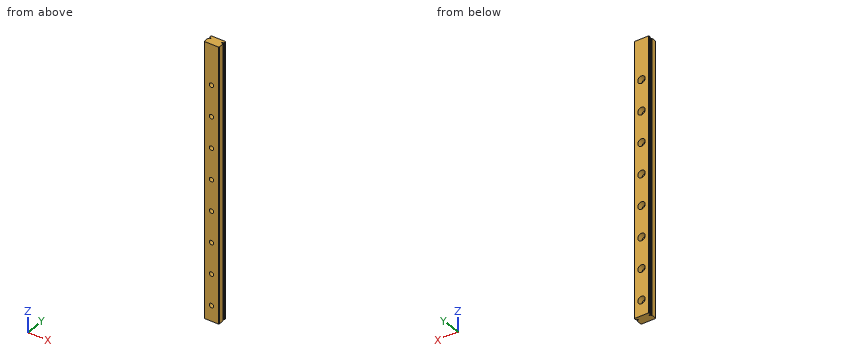
from build123d import *

# Parameters (mm, degrees)
BOSS_EXTRUDE1_DEPTH = 220
SKETCH2_R           = 3
CUT_EXTRUDE1_DEPTH  = 4.5
SKETCH3_R           = 1.75
CUT_EXTRUDE2_DEPTH  = 221.127803787
LPATTERN1_COUNT     = 8
LPATTERN1_PITCH     = 25


with BuildPart() as part:
    # Sketch1 → Boss-Extrude1 (new body)
    with BuildSketch(Plane.XY):
        with BuildLine():
            Line((6, -3.5), (6, 0.368911094))
            ThreePointArc((6, 0.368911094), (5.63354293, 0.61854293), (5.383911094, 0.985))
            Line((5.383911094, 0.985), (4.92112495, 0.985))
            ThreePointArc((4.92112495, 0.985), (4.265, 1.46), (4.92112495, 1.935))
            Line((4.92112495, 1.935), (5.383911094, 1.935))
            ThreePointArc((5.383911094, 1.935), (5.63354293, 2.30145707), (6, 2.551088906))
            Line((6, 2.551088906), (6, 3.5))
            Line((6, 3.5), (5.5, 4))
            Line((5.5, 4), (-5.5, 4))
            Line((-5.5, 4), (-6, 3.5))
            Line((-6, 3.5), (-6, 2.551088906))
            ThreePointArc((-6, 2.551088906), (-5.63354293, 2.30145707), (-5.383911094, 1.935))
            Line((-5.383911094, 1.935), (-4.92112495, 1.935))
            ThreePointArc((-4.92112495, 1.935), (-4.265, 1.46), (-4.92112495, 0.985))
            Line((-4.92112495, 0.985), (-5.383911094, 0.985))
            ThreePointArc((-5.383911094, 0.985), (-5.63354293, 0.61854293), (-6, 0.368911094))
            Line((-6, 0.368911094), (-6, -3.5))
            Line((-6, -3.5), (-5.5, -4))
            Line((-5.5, -4), (5.5, -4))
            Line((5.5, -4), (6, -3.5))
        make_face()
    extrude(amount=BOSS_EXTRUDE1_DEPTH)

    # Sketch2 → Cut-Extrude1 (cut)
    with BuildSketch(Plane(origin=(0, 4, 0), x_dir=(1, 0, 0), z_dir=(0, 1, 0))):
        with Locations(Location((0, -12.5, 0), (0, 0, 180))):
            Circle(SKETCH2_R)
    cut_extrude1 = extrude(amount=-CUT_EXTRUDE1_DEPTH, mode=Mode.SUBTRACT)

    # Sketch3 → Cut-Extrude2 (cut, through all)
    with BuildSketch(Plane(origin=(0, -0.5, 0), x_dir=(1, 0, 0), z_dir=(0, 1, 0))):
        with Locations(Location((0, -12.5, 0), (0, 0, 180))):
            Circle(SKETCH3_R)
    cut_extrude2 = extrude(amount=-CUT_EXTRUDE2_DEPTH, mode=Mode.SUBTRACT)

    # LPattern1: Cut-Extrude1, Cut-Extrude2 ×8
    with Locations(*[(0, 0, i * LPATTERN1_PITCH) for i in range(1, LPATTERN1_COUNT)]):
        add(cut_extrude1, mode=Mode.SUBTRACT)
        add(cut_extrude2, mode=Mode.SUBTRACT)


solid = part.part
Could you check a few things on this model? Use its own coordinates, in mm. Give positions to 0.01 mm unless a question says otherwise; leave off trailing zeros. Order: outer loops, then holes, each group sorted by start corner. A loop starts at its lowest first (then second) coordinate and runs counter-clockwise, first axis right, second up. Notation, with made-up numbers: (18.5, -31) - (45.5, -31) arc R36 cw to (45.5, 3) - close; hole circle Ø1 at (44.25, -10). An arc over 180 degrees is marked (long way). One line per item, written item: value. Start each with the question number.
1. For P1, Ø5.5, axis at x = 0, z = 12.5, coming from the -Y side; P2, Ø5.5, axis at x = 0, z = 162.5, coming from the +Y side, each with a flat end and sliding along its axis, tell me the tip position at first contact or that it passes through.
2. Imagine slicing it at B-B on z = 149. List the corners of the cut face in (x, y) for me (3 decimals).
3. If I drill on probe 1 along Y at (x, z) = (-5, 135.5) (3 decimals); probe 2 along X at (y, z) = (2.2, 187.5); probe 3 along X at (y, z) = (-3.15, 162.5), over which ranges is the centre line in solid material (lowest first)?
4. Imagine slicing it at A-A on y = -2. Give the number of separate pieces and of enclosed holes in the cut face, plus the area to 3 significant figures.
Values:
1. P1: y = -4
1. P2: y = -0.5
2. outline: (-6, -3.5) - (-5.5, -4) - (5.5, -4) - (6, -3.5) - (6, 0.369) arc R1.19 cw to (5.384, 0.985) - (4.921, 0.985) arc R0.5 cw (long way) to (4.921, 1.935) - (5.384, 1.935) arc R1.19 cw to (6, 2.551) - (6, 3.5) - (5.5, 4) - (-5.5, 4) - (-6, 3.5) - (-6, 2.551) arc R1.19 cw to (-5.384, 1.935) - (-4.921, 1.935) arc R0.5 cw (long way) to (-4.921, 0.985) - (-5.384, 0.985) arc R1.19 cw to (-6, 0.369) - close
3. probe 1: -4 to 0.985, 1.935 to 4
3. probe 2: -5.54 to -3, 3 to 5.54
3. probe 3: -6 to -1.75, 1.75 to 6
4. separate pieces: 1
4. enclosed holes: 8
4. area: 2,560 mm²
